Read the model definition and answer for the solid it produces. Units are mm, in the model's axes. A direction names the side the tool comes from. Give positions to 0.01 mm unless a question says otherwise; leave off trailing zeros. Order: outer loops, then holes, each group sorted by start corner. A loop starts at its lowest first (then second) coordinate and runs counter-clockwise, first axis right, second up. Notation, with made-up numbers: (80.25, 89) -> (88.25, 89) arc R6 ccw to (88.25, 96) -> close; hole circle Ø9 at (-2.5, 63). An arc over 180 degrees is marked (long way). Use one line per item in the form item = value.
```python
from build123d import *

# Parameters (mm, degrees)
F0_R            = 25
F1_DEPTH        = 91
F2_R            = 23.5
F3_DEPTH        = 2.15
F4_R            = 25
F5_DEPTH        = 3.25
F6_SIZE         = 1
F7_R            = 20
F8_DEPTH        = 8
F9_R            = 18
F10_DEPTH       = 30
F11_SIZE        = 1
F12_SIZE        = 2
F14_D           = 6
F14_DEPTH       = 60
F14_CBORE_D     = 12
F14_CBORE_DEPTH = 12
F14_TIP         = 1.8025818571
F17_D           = 6


with BuildPart() as f1:
    # F0 (on Top) → F1 (new body)
    with BuildSketch(Plane.XY):
        Circle(F0_R)
    extrude(amount=F1_DEPTH)

    # F2 (on face) → F3 (join)
    with BuildSketch(Plane.XY.offset(91)):
        Circle(F2_R)
    extrude(amount=F3_DEPTH)

    # F4 (on face) → F5 (join)
    with BuildSketch(Plane.XY.offset(93.15)):
        Circle(F4_R)
    extrude(amount=F5_DEPTH)

    # F6
    f6_edges = [f1.edges().sort_by_distance(p)[0] for p in [
        (-25, 0, 96.4),
    ]]
    chamfer(f6_edges, length=F6_SIZE)

    # F7 (on face) → F8 (join)
    with BuildSketch(Plane(origin=(0, 0, 0), x_dir=(1, 0, 0), z_dir=(0, 0, -1))):
        Circle(F7_R)
    extrude(amount=F8_DEPTH)

    # F9 (on face) → F10 (join)
    with BuildSketch(Plane(origin=(0, 0, -8), x_dir=(1, 0, 0), z_dir=(0, 0, -1))):
        Circle(F9_R)
    extrude(amount=F10_DEPTH)

    # F11
    f11_edges = [f1.edges().sort_by_distance(p)[0] for p in [
        (-25, 0, 0),
        (-20, 0, -8),
    ]]
    chamfer(f11_edges, length=F11_SIZE)

    # F12
    f12_edges = [f1.edges().sort_by_distance(p)[0] for p in [
        (-18, 0, -38),
    ]]
    chamfer(f12_edges, length=F12_SIZE)

    # F14
    with Locations(Plane.XY.offset(96.4)):
        with Locations((0, 0)):
            CounterBoreHole(F14_D / 2, F14_CBORE_D / 2, F14_CBORE_DEPTH, depth=F14_DEPTH)
            with Locations((0, 0, -(F14_DEPTH + F14_TIP / 2))):  # 118° drill point
                Cone(0, F14_D / 2, F14_TIP, mode=Mode.SUBTRACT)

    # F17 (through all)
    with Locations(Plane.XZ.offset(25)):
        with Locations((0, 50.4)):
            Hole(F17_D / 2)


solid = f1.part
```
Item 1: Determine the mould class of faces 4 (the cylindrical face through (23.846, 7.509, 45.37)), 5 (the conical face through (0.24, -0.46, 34.91)), 6 (the flat face through (-17, -17, 93.15)) for opening direction Y: +Y half, -Y half, draft (parallel to the pull), parting line (faces both ways), or undercut.
Checks:
face_4 = parting line
face_5 = undercut
face_6 = draft
Item 2: Straight lines are drawn through the part: L1, parallel to X at y = -7, z = 50; L2, parallel to Y at x = 0, z = 92.25; L3, parallel to Y at x = 0, z = 40. For each, find the intervals that lie inside material, in ascending order. Write a range as from..to.
Checks:
L1 = -24..-2.97, 2.97..24
L2 = -23.5..-6, 6..23.5
L3 = -25..-3, 3..25
Item 3: The part is cut by section A-A on z = 78. Give the vertices of the cut face in (x, y).
Checks:
outline = circle Ø50 at (0, 0); hole circle Ø6 at (0, 0)
Item 4: Which of the six approach directions +Z, -Z, +X, -X, +Y, -Y give full straight-line access (tool end or side, diameter ignored) to faces 1 (the cylindrical face through (-6, 0, 90)), 2 (the flat face through (-5, 20, 0)), 3 (the flat face through (-17, -17, 91))?
Checks:
face_1 = +Z
face_2 = -Z
face_3 = none
Item 5: Given pin 1 Ø5.5 at (x, y) = (0, 0) entering from +Z; pin 2 Ø2 at (y, z) = (-8.5, 30) entering from +X; pin 3 Ø5 at (x, y) = (0, 0) entering from +Z, each flat-ended and moving along its own axis, determine where each tip first touches the part or whether it passes through.
Checks:
pin_1 = 36.25
pin_2 = 23.85
pin_3 = 36.1
Item 6: The part is cut by section B-B on x = -1.5. State how many separate pieces and enclosed holes the cut face has, and give its area (3 significant figures).
Checks:
separate_pieces = 3
enclosed_holes = 0
area = 5,570 mm²
